Could you check a few things on this drawing? It's one solid part, dimensions in mm from its lowest x, y, z. Coordinates: 2 decimals unless noted, no trailing zeros. Write each loop counter-clockwise with the first axis right and the second up, starting at its lowest first coordinate (ties: lowest second). Pieces come first, ordered by that corner, then holes.
Item 1: Please list where these lines run through material, in increasing order: line 1 (Z direction, x = 4.4, y = 7); line 2 (Y direction, x = 3.4, z = 3) (1 decimal); line 3 (Y direction, x = 4.85, z = 7).
Item 2: I want a section at A-A (x = 5). Please give me the cut outline in (y, z).
Item 3: I'm going to push flat-ended pins straight in: P1, Ø2, axis at y = 4, z = 7, coming from the +X side; P2, Ø1.5, axis at x = 1, z = 10, coming from the +Y side. Where does each tip first touch, or does it pass through?
Item 4: If we mould it in two halves opening along Z, with no side actions, what happens to the marked faces 1, 2, 3 and 4? For each: pulls with the +Z half, pulls with the -Z half, needs draft (parallel to the pull), parting line crosses it, or undercut.
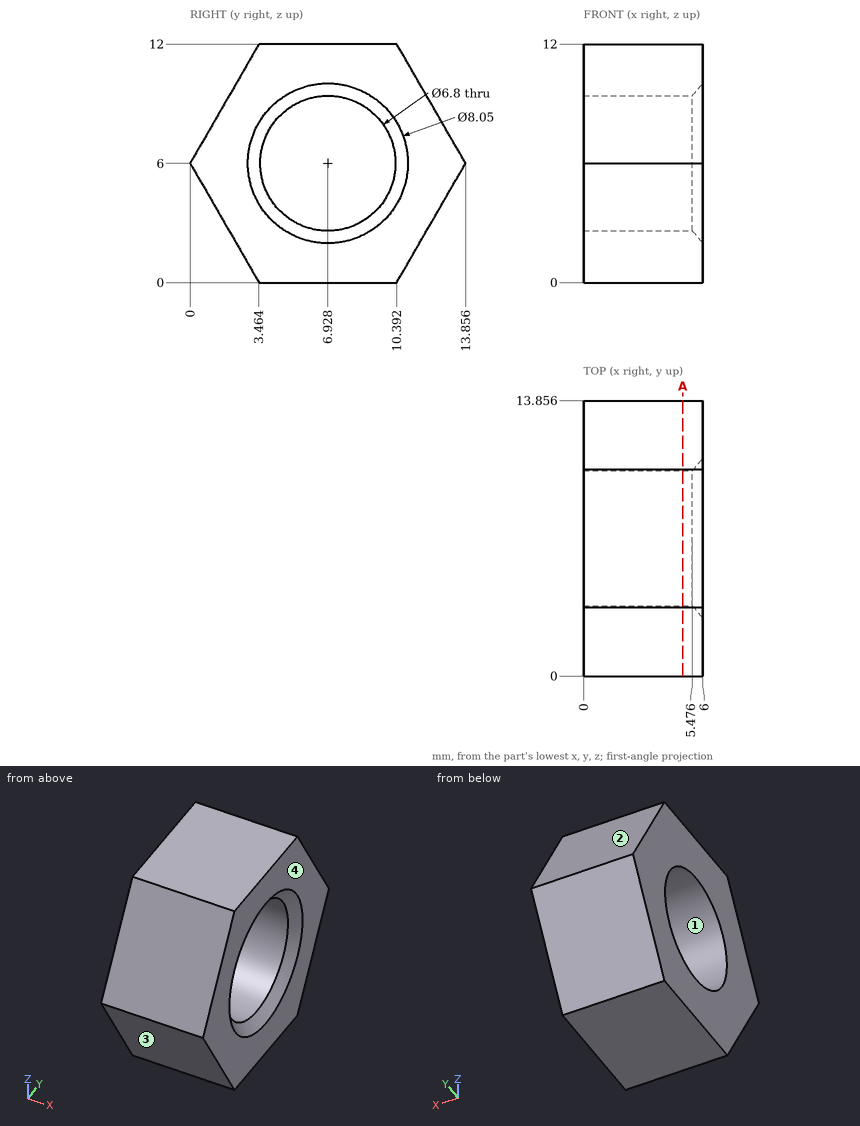
Answer:
1. line 1: z = 0 to 2.6, 9.4 to 12
1. line 2: y = 1.7 to 5.3, 8.5 to 12.1
1. line 3: y = 0.58 to 3.68, 10.18 to 13.28
2. outline: (0, 6) - (3.46, 0) - (10.39, 0) - (13.86, 6) - (10.39, 12) - (3.46, 12) - close; hole circle Ø6.8 at (6.93, 6)
3. P1: stops at x = 6
3. P2: stops at y = 11.98
4. face 1: undercut
4. face 2: pulls with the +Z half
4. face 3: pulls with the -Z half
4. face 4: needs draft
